Input: part model. Units: mm. Frame: model coordinates. Coordinates: 2 decimals unless noted, no trailing zeros.
1) Section query A-A (y = 4.75). State how many separate pieces and enclosed holes the cut face has, then the cut area to 3 significant figures.
2) Pin query (flat end, axial travel): pin 1 Ø0.5 at (x, z) = (7, 29) entering from -Y; pin 2 Ø2 at (x, z) = (162.5, 21.5) entering from -Y. Return the tip coordinate at first contact, or that it passes through.
3) Line query: L1, parallel to Y at x = 62, z = 16; L2, parallel to Y at x = 147.5, z = 27. Output: solid intervals per line, ascending.
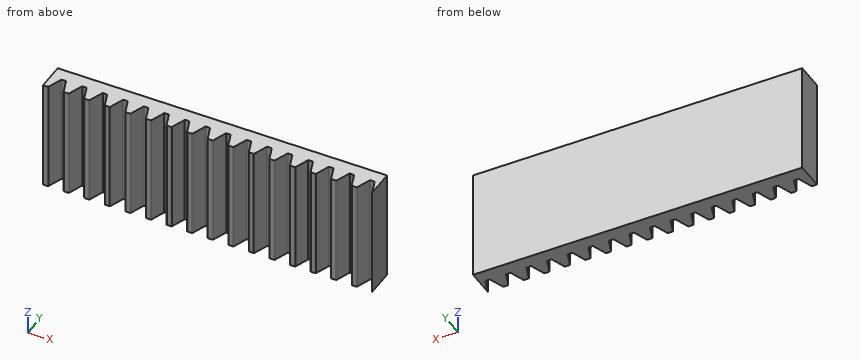
from build123d import *

# Parameters (mm, degrees)
BOSS_EXTRUDE1_DEPTH = 60
FILLET1_R           = 0.5
LPATTERN1_COUNT     = 8
LPATTERN1_PITCH     = 22.2470475
FILLET2_R           = 0.5


with BuildPart() as part:
    # Sketch1 → Boss-Extrude1 (new body)
    with BuildSketch(Plane.XY):
        Polygon((0, 0), (2.8, 0), (5.711761874, 8), (8.211761874, 8), (11.123523748, 0), (13.923523748, 0), (16.835285622, 8), (19.335285622, 8), (22.247047497, 0), (22.247047497, 15), (0, 15), align=None)
    extrude(amount=BOSS_EXTRUDE1_DEPTH)

    # Fillet1
    fillet1_edges = [part.edges().sort_by_distance(p)[0] for p in [
        (19.335285622, 8, 30),
        (16.835285622, 8, 30),
        (13.923523748, 0, 30),
        (11.123523748, 0, 30),
        (8.211761874, 8, 30),
        (5.711761874, 8, 30),
        (2.8, 0, 30),
    ]]
    fillet(fillet1_edges, radius=FILLET1_R)


with BuildPart() as lpattern1_1:
    # LPattern1: pattern copy
    add(part.part.moved(Location(Vector(1, 0, 0) * (1 * LPATTERN1_PITCH))))


with BuildPart() as lpattern1_2:
    # LPattern1: pattern copy
    add(part.part.moved(Location(Vector(1, 0, 0) * (2 * LPATTERN1_PITCH))))


with BuildPart() as lpattern1_3:
    # LPattern1: pattern copy
    add(part.part.moved(Location(Vector(1, 0, 0) * (3 * LPATTERN1_PITCH))))


with BuildPart() as lpattern1_4:
    # LPattern1: pattern copy
    add(part.part.moved(Location(Vector(1, 0, 0) * (4 * LPATTERN1_PITCH))))


with BuildPart() as lpattern1_5:
    # LPattern1: pattern copy
    add(part.part.moved(Location(Vector(1, 0, 0) * (5 * LPATTERN1_PITCH))))


with BuildPart() as lpattern1_6:
    # LPattern1: pattern copy
    add(part.part.moved(Location(Vector(1, 0, 0) * (6 * LPATTERN1_PITCH))))


with BuildPart() as lpattern1_7:
    # LPattern1: pattern copy
    add(part.part.moved(Location(Vector(1, 0, 0) * (7 * LPATTERN1_PITCH))))


with BuildPart() as part_1:
    add(part.part)

    # Combine1: union LPattern1_1, LPattern1_2, LPattern1_3, LPattern1_4, LPattern1_5, LPattern1_6, LPattern1_7
    add(lpattern1_1.part)
    add(lpattern1_2.part)
    add(lpattern1_3.part)
    add(lpattern1_4.part)
    add(lpattern1_5.part)
    add(lpattern1_6.part)
    add(lpattern1_7.part)

    # Fillet2
    fillet2_edges = [part_1.edges().sort_by_distance(p)[0] for p in [
        (44.494094997, 0, 30),
        (66.741142497, 0, 30),
        (88.988189997, 0, 30),
        (22.247047497, 0, 30),
    ]]
    fillet(fillet2_edges, radius=FILLET2_R)


solid = part_1.part
Answer:
1. separate pieces: 17
1. enclosed holes: 0
1. area: 6,010 mm2
2. pin 1: stops at y = 8
2. pin 2: stops at y = 7.91
3. L1: y = 8 to 15
3. L2: y = 0.27 to 15
